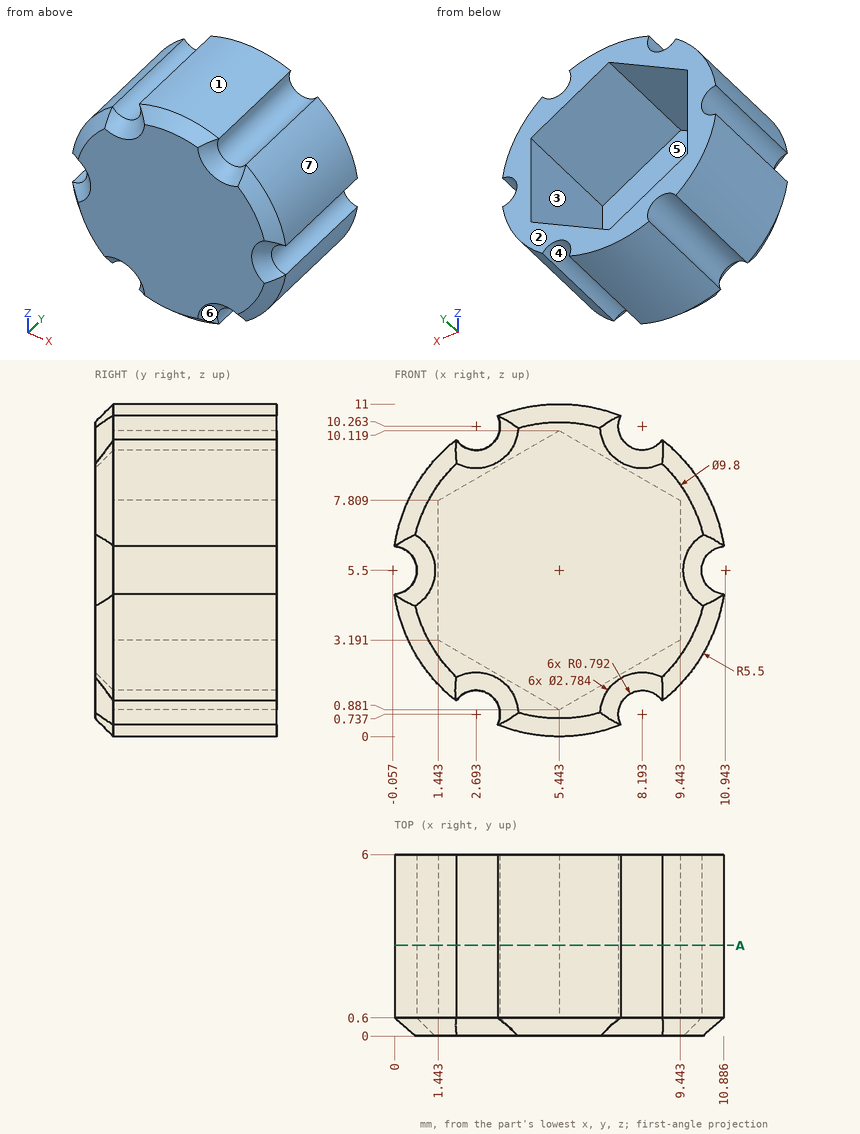
Geometry: see drawing. Coordinates: mm, zero at the bounding-box minimum. A direction names the side the tool comes from. Give positions to 0.01 mm unless a question says otherwise; leave off trailing zeros. Order: outer loops, then holes, each group sorted by start corner. A loop starts at its lowest first (then second) coordinate and runs counter-clockwise, first axis right, second up. Notation, with made-up numbers: (-19, -21.5) - (-13, -21.5) arc R17 cw to (-13, -12.5) - close; hole circle Ø10 at (-7, 28). An arc over 180 degrees is marked (long way). Write each question's results on one line, items separated by ' | '.
Item 1: Draft query along Z for the marked faces 1, 2, 3 and 4. Return one class per face: released by +Z, released by -Z, zero draft, split by the parting line, or undercut.
A:
face 1: released by +Z | face 2: zero draft | face 3: undercut | face 4: undercut
Item 2: Section A-A (y = 3). Return loops of the section in (x, z) (1 decimal).
A:
outline: (0, 4.7) arc R5.5 ccw to (2, 1.2) arc R0.8 cw to (3.4, 0.4) arc R5.5 ccw to (7.5, 0.4) arc R0.8 cw to (8.8, 1.2) arc R5.5 ccw to (10.9, 4.7) arc R0.8 cw to (10.9, 6.3) arc R5.5 ccw to (8.8, 9.8) arc R0.8 cw to (7.5, 10.6) arc R5.5 ccw to (3.4, 10.6) arc R0.8 cw to (2, 9.8) arc R5.5 ccw to (0, 6.3) arc R0.8 cw to start; hole (1.4, 3.2) - (5.4, 0.9) - (9.4, 3.2) - (9.4, 7.8) - (5.4, 10.1) - (1.4, 7.8) - close
Item 3: Material intervals for line 1 along Y through (x, z) = (3.75, 6.75); line 2 along X through (y, z) = (1, 5.5) (1 decimal); line 3 along Z through (x, y) = (8.5, 1.5) (1 decimal), sorted ascending.
A:
line 1: y = 0 to 0.6 | line 2: x = 0.7 to 1.4, 9.4 to 10.2 | line 3: z = 1.5 to 2.6, 8.4 to 9.5
Item 4: Access query for the marked faces 5, 6 and 7. Directions: +Z, -Z, +X, -X, +Y, -Y. A direction counts if a zero-diameter tool reaches every point of the face in a straight line with its end or side. Return the directions, or none.
A:
face 5: +Y | face 6: -Y | face 7: +Z, +X, +Y, -Y
Item 5: Contact query for a flat-ended pin moving along its axis: pin 1 Ø4 at (x, z) = (3.5, 5.5) entering from +Y. Output: stop coordinate, or through.
A:
pin 1: stops at y = 0.6
